Input: part model. Units: mm. Frame: model coordinates. A direction names the side the tool comes from. Give positions to 0.01 mm unless a question says otherwise; leave off trailing zeros. Loops run counter-clockwise (first coordinate to the right, second up) from the corner with the lowest first, then second, coordinate; pieces in that order, holes last. Notation, with made-up numbers: (70, -38.75) - (103, -38.75) arc R17 ccw to (103, -25.75) - close; hole circle Ø1 at (39.5, 64.25). An arc over 180 degrees is marked (long way). Answer as a JSON object with one key per item and string values.
Autodesk Inventor part; units mm, degrees
ref_plane "YZ Plane" through (0, 0, 0) normal (1, 0, 0) x (0, 1, 0)
ref_plane "XZ Plane" through (0, 0, 0) normal (0, 1, 0) x (-1, 0, 0)
ref_plane "XY Plane" through (0, 0, 0) normal (0, 0, 1) x (1, 0, 0)
sketch "Sketch1" plane through (0, 0, 0) normal (1, 0, 0) x (0, 1, 0)
  line L0 (-3.675, 8) -> (3.675, 8)
  line L1 (3.675, 8) -> (3.675, -8)
  line L2 (3.675, -8) -> (-3.675, -8)
  line L3 (-3.675, -8) -> (-3.675, 8)
  line L4 (-3.675, 8) -> (3.675, -8) construction
  line L5 (3.675, 8) -> (-3.675, -8) construction
  line L6 (4.175, -8.5) -> (4.175, 8.5)
  line L7 (4.175, 8.5) -> (-4.175, 8.5)
  line L8 (-4.175, 8.5) -> (-4.175, -8.5)
  line L9 (-4.175, -8.5) -> (4.175, -8.5)
  point P0 (0, 0)
  dimension "d0" = 7.35
  dimension "d1" = 16
  dimension "d2" = 0.5
extrude "Extrusion1" add sketch "Sketch1" along normal blind 28
fillet "Fillet1" radius 1 8 edges at (14, -3.675, -8) (14, 3.675, -8) (14, 4.175, -8.5) (14, 4.175, 8.5) (14, 3.675, 8) (14, -4.175, -8.5) (14, -3.675, 8) (14, -4.175, 8.5)
properties part number "HeatShrink" material "Rubber, Silicone"
Item 1: Cut plane A-A (y = 0.5). Return loops of the section in (x, z), then the cut area to 3 significant figures.
Geometry check:
{"outline": "(0, -8.5) - (28, -8.5) - (28, -8) - (0, -8) - close; (0, 8) - (28, 8) - (28, 8.5) - (0, 8.5) - close", "area": "28.0 mm2"}
Item 2: Material intervals for line 1 (Z direction, x = 17, y = -1.5); line 2 (Y direction, x = 20.25, z = 0) (3 decimals); line 3 (Y direction, x = 10.25, z = -7.25) (3 decimals), sorted ascending. Write a range as [from, to].
Geometry check:
{"line 1": "z = [-8.5, -8], [8, 8.5]", "line 2": "y = [-4.175, -3.675], [3.675, 4.175]", "line 3": "y = [-4.175, -3.643], [3.643, 4.175]"}
Item 3: Cut plane C-C (x = 20). Return loops of the section in (y, z) (3 decimals).
Geometry check:
{"outline": "(-4.175, -7.5) arc R1 ccw to (-3.175, -8.5) - (3.175, -8.5) arc R1 ccw to (4.175, -7.5) - (4.175, 7.5) arc R1 ccw to (3.175, 8.5) - (-3.175, 8.5) arc R1 ccw to (-4.175, 7.5) - close; hole (-3.675, -7) arc R1 ccw to (-2.675, -8) - (2.675, -8) arc R1 ccw to (3.675, -7) - (3.675, 7) arc R1 ccw to (2.675, 8) - (-2.675, 8) arc R1 ccw to (-3.675, 7) - close"}
Item 4: Mould query, pull axis Y, two halves, no side actions, for faces 3 (the face through (14.196, -3.374, 7.715)), 4 (the face through (14, 4.175, 0)), 5 (the face through (14.2, -3.89, -8.2)), 6 (the face through (14, 0, 8)). Classes: released by +Y, released by -Y, zero draft, split by the parting line, or undercut.
Geometry check:
{"face 3": "undercut", "face 4": "released by +Y", "face 5": "released by -Y", "face 6": "undercut"}
Item 5: Cut plane B-B (z = 4.25). Return loops of the section in (x, y) (3 decimals).
Geometry check:
{"outline": "(0, -4.175) - (28, -4.175) - (28, -3.675) - (0, -3.675) - close; (0, 3.675) - (28, 3.675) - (28, 4.175) - (0, 4.175) - close"}
Item 6: Access query for faces 1 (the face through (14.2, 3.39, 7.7)), 2 (the face through (14.196, 3.874, -8.215)). Directions: +Z, -Z, +X, -X, +Y, -Y. A direction counts if a zero-diameter tool reaches every point of the face in a straight line with its end or side. Return the directions, or none.
Geometry check:
{"face 1": "+X, -X", "face 2": "-Z, +X, -X, +Y"}
